Source: CAD feature listing. Evaluate the final solid. Frame: model axes, mm. Face numbers are marked on the shaded views. Give positions to 0.01 mm unless a question says otherwise; leave off trailing zeros.
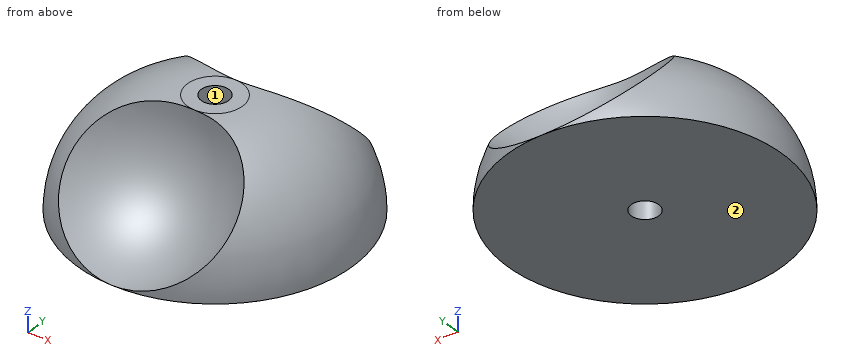
from build123d import *

# Parameters (mm, degrees)
SKETCH1_R           = 5
BOSS_EXTRUDE1_DEPTH = 4
FILLET1_R           = 4
SKETCH3_R           = 0.5
CUT_EXTRUDE1_DEPTH  = 9.124038577


with BuildPart() as part:
    # Sketch1 → Boss-Extrude1 (new body)
    with BuildSketch(Plane.XY):
        Circle(SKETCH1_R)
    extrude(amount=BOSS_EXTRUDE1_DEPTH)

    # Fillet1
    fillet1_edges = [part.edges().sort_by_distance(p)[0] for p in [
        (-5, 0, 4),
    ]]
    fillet(fillet1_edges, radius=FILLET1_R - 0.0001)  # a hair under: the kernel refuses the full size

    # Sketch2 → Cut-Revolve2 (revolve, cut)
    with BuildSketch(Plane(origin=(0, 0, 0), x_dir=(0, 0, -1), z_dir=(1, 0, 0))):
        with BuildLine():
            Line((0, 5), (-8, 5))
            ThreePointArc((-8, 5), (-4, 1), (0, 5))
        make_face()
    cut_revolve2 = revolve(axis=Axis((0, 5, 0), (0, 0, 1)), mode=Mode.SUBTRACT)

    # Mirror1: Cut-Revolve2 across plane
    add(cut_revolve2.mirror(Plane.ZX), mode=Mode.SUBTRACT)

    # Sketch3 → Cut-Extrude1 (cut, through all)
    with BuildSketch(Plane(origin=(0, 0, 0), x_dir=(-1, 0, 0), z_dir=(0, 0, -1))):
        Circle(SKETCH3_R)
    extrude(amount=-CUT_EXTRUDE1_DEPTH, mode=Mode.SUBTRACT)


solid = part.part
1) Pull-direction query (Y, two-part tool) for the marked faces 1 and 2; classes: released by +Y, released by -Y, zero draft, split by the parting line, or undercut.
Checks:
face 1: undercut
face 2: zero draft
2) Contact query for flat-ended pins moving along their axis: P1, Ø3, axis at x = 1, y = 2.5, coming from the +Z side; P2, Ø2, axis at y = 3, z = 3, coming from the -X side; P3, Ø2, axis at x = 0, z = 2, coming from the -Y side. Output: stop coordinate, or through.
Checks:
P1: stops at z = 3.99
P2: stops at x = -3.62
P3: stops at y = -2.35
3) Ray query, probe 1 along Y at (x, z) = (0, 2.45); probe 2 along Y at (x, z) = (0, 1.3); probe 3 along Z at (x, y) = (2.5, -3). Return the intervals inside material, ascending.
Checks:
probe 1: y = -1.31 to -0.5, 0.5 to 1.31
probe 2: y = -2.05 to -0.5, 0.5 to 2.05
probe 3: z = 0 to 1.6
